from build123d import *

# Parameters (mm, degrees)
BOSS_EXTRUDE1_DEPTH = 50.8
CUT_EXTRUDE1_DEPTH  = 50.8
SKETCH5_R           = 2.032
BOSS_EXTRUDE2_DEPTH = 4.572
SKETCH8_R           = 2.413
BOSS_EXTRUDE3_DEPTH = 37.846
FILLET1_R           = 12.7


with BuildPart() as part:
    # Sketch1 → Boss-Extrude1 (new body)
    with BuildSketch(Plane(origin=(0, 0, 0), x_dir=(1, 0, 0), z_dir=(0, 1, 0))):
        Polygon((-0.528142549, -56.463008639), (-0.528142549, -28.015008639), (-6.878142549, -28.015008639), (-6.878142549, -62.813008639), (12.044857451, -62.813008639), (12.044857451, -56.463008639), align=None)
        Polygon((-0.528142549, -28.015008639), (-0.528142549, 0.432991361), (12.044857451, 0.432991361), (12.044857451, 6.782991361), (-6.878142549, 6.782991361), (-6.878142549, -28.015008639), align=None)
        Polygon((12.044857451, 6.782991361), (12.044857451, 0.432991361), (24.617857451, 0.432991361), (24.617857451, -28.015008639), (30.967857451, -28.015008639), (30.967857451, 6.782991361), align=None)
        Polygon((24.617857451, -56.463008639), (12.044857451, -56.463008639), (12.044857451, -62.813008639), (30.967857451, -62.813008639), (30.967857451, -28.015008639), (24.617857451, -28.015008639), align=None)
    extrude(amount=BOSS_EXTRUDE1_DEPTH)

    # Sketch3 → Cut-Extrude1 (cut)
    with BuildSketch(Plane.XY.offset(62.813008639)):
        Polygon((5.694857451, 29.21), (12.044857451, 29.21), (18.394857451, 29.21), (18.394857451, 50.8), (5.694857451, 50.8), align=None)
    extrude(amount=-CUT_EXTRUDE1_DEPTH, mode=Mode.SUBTRACT)

    # Sketch5 → Boss-Extrude2 (add)
    with BuildSketch(Plane(origin=(0, 1.016, 0), x_dir=(1, 0, 0), z_dir=(0, 1, 0))):
        Polygon((30.967857451, -62.813008639), (12.044857451, -62.813008639), (-6.878142549, -62.813008639), (-6.878142549, -75.513008639), (30.967857451, -75.513008639), align=None)
        with Locations(Location((5.694857451, -70.332821617, 0), (0, 0, 270))):
            Circle(SKETCH5_R, mode=Mode.SUBTRACT)
        with Locations(Location((18.394857451, -70.332821617, 0), (0, 0, 270))):
            Circle(SKETCH5_R, mode=Mode.SUBTRACT)
    extrude(amount=BOSS_EXTRUDE2_DEPTH)

    # Sketch8 → Boss-Extrude3 (add)
    with BuildSketch(Plane(origin=(30.967857451, 0, 0), x_dir=(0, 0, -1), z_dir=(1, 0, 0))):
        Polygon((6.782991361, 0), (15.926991361, 0), (23.037514196, 0), (23.037514196, 16.864021844), (6.782991361, 33.63258694), align=None)
        with Locations((15.926991361, 4.445)):
            Circle(SKETCH8_R, mode=Mode.SUBTRACT)
    extrude(amount=-BOSS_EXTRUDE3_DEPTH)

    # Fillet1
    fillet1_edges = [part.edges().sort_by_distance(p)[0] for p in [
        (12.044857451, 33.63258694, -6.782991361),
        (12.044857451, 16.864021844, -23.037514196),
    ]]
    fillet(fillet1_edges, radius=FILLET1_R)


solid = part.part
The listing builds one solid part. Answer for the finished solid, in the listing's coordinates (mm). A direction names the side the tool comes from. Give positions to 0.01 mm unless a question says otherwise; leave off trailing zeros. Write each loop counter-clockwise with the first axis right and the second up, starting at its lowest first coordinate (ties: lowest second). Pieces come first, ordered by that corner, then holes. Notation, with made-up numbers: (-21.75, 63) -> (0.25, 63) arc R19 ccw to (0.25, 73) -> close; hole circle Ø9 at (2.5, 54). An arc over 180 degrees is marked (long way). One line per question, with ' | ' between items. Start each with the question number.
1. Section B-B (z = 49) is taken. Determine the outline of the cut face in (x, y), plus the area to 3 significant figures.
2. Section D-D (z = 70.5) is taken. Determine the outline of the cut face in (x, y).
3. For faces 4 (the flat face through (12, 25, -0.433)), 5 (the flat face through (30.968, 26, 27)), 6 (the flat face through (12, 5.588, 69)), 7 (the flat face through (12, 1.016, 69)), 8 (the flat face through (12, 29.21, 60)), determine the directions among +Z, -Z, +X, -X, +Y, -Y from which every point of the face is accessible in a straight line to the end or side of a thin tool.
4. Section A-A (y = 8) is taken. Determine the outline of the cut face in (x, z).
5. Section C-C (x = 22.5) is taken. Determine the outline of the cut face in (y, z) (3 decimals), plus the area to 3 significant figures.
6. Given pin 1 Ø3.5 at (x, z) = (5.69, 70.33) entering from -Y; pin 2 Ø10 at (x, z) = (13.5, 69) entering from +Y; pin 3 Ø0.8 at (x, y) = (14.5, 0.5) entering from +Z; pin 4 Ø2 at (x, y) = (0, 18) entering from -Z, each flat-ended and moving along its own axis, determine where each tip first touches the part or whether it passes through.
7. For a pull along Z with two mould halves and no side action, classify faces 1 (the flat face through (12, 19, 56.463)), 2 (the flat face through (18.395, 40, 60)), 3 (the cylindrical face through (11.78, 16.551, -22.082)) as pulls with the +Z half, pulls with the -Z half, needs draft (parallel to the pull), parting line crosses it, or undercut.
8. Find the intervals of material crossed by probe 1 along X at (y, z) = (11, 0.5); probe 2 along Z at (x, y) = (7, 8); probe 3 along Y at (x, z) = (17, 58.5), in increasing order.
Response values:
1) outline: (-6.88, 0) -> (-0.53, 0) -> (-0.53, 50.8) -> (-6.88, 50.8) -> close; (24.62, 0) -> (30.97, 0) -> (30.97, 50.8) -> (24.62, 50.8) -> close | area: 645 mm2
2) outline: (-6.88, 1.02) -> (3.67, 1.02) -> (3.67, 5.59) -> (-6.88, 5.59) -> close; (7.72, 1.02) -> (16.37, 1.02) -> (16.37, 5.59) -> (7.72, 5.59) -> close; (20.42, 1.02) -> (30.97, 1.02) -> (30.97, 5.59) -> (20.42, 5.59) -> close
3) face 4: +Y, -Y | face 5: +Z, -Z, +X, +Y, -Y | face 6: +Z, +X, -X, +Y | face 7: +Z, +X, -X, -Y | face 8: +Z, +Y
4) outline: (-6.88, -23.04) -> (30.97, -23.04) -> (30.97, 62.81) -> (-6.88, 62.81) -> close; hole (-0.53, -0.43) -> (24.62, -0.43) -> (24.62, 56.46) -> (-0.53, 56.46) -> close
5) outline: (0, -23.038) -> (11.719, -23.038) arc R12.7 ccw to (20.558, -19.456) -> (29.938, -10.364) arc R12.7 cw to (38.778, -6.783) -> (50.8, -6.783) -> (50.8, -0.433) -> (0, -0.433) -> close; (0, 56.463) -> (50.8, 56.463) -> (50.8, 62.813) -> (5.588, 62.813) -> (5.588, 75.513) -> (1.016, 75.513) -> (1.016, 62.813) -> (0, 62.813) -> close; hole circle Ø4.826 at (4.445, -15.927) | area: 1,100 mm2
6) pin 1: through | pin 2: y = 5.59 | pin 3: z = 62.81 | pin 4: z = -21.89
7) face 1: undercut | face 2: needs draft | face 3: pulls with the -Z half
8) probe 1: -6.88 to -0.53, 24.62 to 30.97 | probe 2: -23.04 to -0.43, 56.46 to 62.81 | probe 3: 0 to 29.21
